Geometry check sheet. Reference: the model listing, model coordinates, mm. A direction names the side the tool comes from. Round coordinates to 2 decimals unless told otherwise and drop trailing zeros. Write each loop counter-clockwise with the first axis right and the second up, starting at its lowest first coordinate (ties: lowest second). Pieces come first, ordered by that corner, then holes. Notation, with made-up numbers: (69.25, 4.5) - (87.25, 4.5) arc R19 ccw to (87.25, 37.5) - close; hole circle Ø9 at (-10.5, 17). An arc over 180 degrees is marked (long way). Return JSON: item names as keys, results as strings.
```python
from build123d import *

# Parameters (mm, degrees)
FILLET1_R   = 0.2
FILLET2_R   = 0.4
HEX_2_DEPTH = 1.6


with BuildPart() as part:
    # BodySke → Base-Revolve (revolve)
    with BuildSketch(Plane.XY):
        Polygon((0, 0), (0, 3.5), (2.8, 3.5), (2.8, 2), (12.41, 2), (12.8, 1.61), (12.8, 0), align=None)
    revolve(axis=Axis((-31.75, 0, 0), (1, 0, 0)))

    # Fillet1
    fillet1_edges = [part.edges().sort_by_distance(p)[0] for p in [
        (2.8, -2, 0),
    ]]
    fillet(fillet1_edges, radius=FILLET1_R)

    # Fillet2
    fillet2_edges = [part.edges().sort_by_distance(p)[0] for p in [
        (0, -3.5, 0),
    ]]
    fillet(fillet2_edges, radius=FILLET2_R)

    # HexSke → Hex 2 (cut)
    with BuildSketch(Plane(origin=(0, 0, 0), x_dir=(0, 0.5, 0.866025404), z_dir=(-1, 0, 0))):
        Polygon((0.866025404, 1.5), (-0.866025404, 1.5), (-1.732050808, 0), (-0.866025404, -1.5), (0.866025404, -1.5), (1.732050808, 0), align=None)
    extrude(amount=-HEX_2_DEPTH, mode=Mode.SUBTRACT)

    # PilotSke → Hex-PreBroach (revolve, cut)
    with BuildSketch(Plane.XY):
        Polygon((0, 1.5), (1.6, 1.5), (1.888675135, 1), (3.3, 1), (3.877350269, 0), (0, 0), align=None)
    revolve(axis=Axis((0, 0, 0), (1, 0, 0)), mode=Mode.SUBTRACT)


solid = part.part
```
(1) Access from +Z, -Z, +X, -X, +Y, -Y to the whole of each face (thin tool, end or side, straight path). Record for faces 4 (the face through (12.8, 0, 0)), 5 (the face through (8, 0, -2)), 6 (the face through (0.789, -1.305, 0.739)).
Response values:
{"face 4": "+Z, -Z, +X, +Y, -Y", "face 5": "+X", "face 6": "-X"}
(2) Section check A-A, the plane x = 5.5. Enter the section's corners in (y, z).
Response values:
{"outline": "circle Ø4 at (0, 0)"}
(3) Gauge pin test, flat ends, axial feed: pin 1 (1 mm diameter, centred on x = 4, z = 0, fed in from +Y); pin 2 (1.6 mm diameter, centred on y = 0, z = 0, fed in from -X); pin 3 (3 mm diameter, centred on x = 7, y = -0.5, fed in from -Z). Record the tip position at first contact, or that the pin passes through.
Response values:
{"pin 1": "stops at y = 2", "pin 2": "stops at x = 3.42", "pin 3": "stops at z = -2"}
(4) Release check for a two-part mould opening along Y. For faces 1 (the face through (0.789, 1.293, 0.761)), 2 (the face through (0, -1.3, -1.3)), 3 (the face through (1.617, 3.233, -1.341)) record: pulls with the +Y half, pulls with the -Y half, needs draft (parallel to the pull), parting line crosses it, or undercut.
Response values:
{"face 1": "undercut", "face 2": "needs draft", "face 3": "parting line crosses it"}
(5) Material ranges on line 1 along Z through (x, y) = (2.4, 0); line 2 along Z through (x, y) = (3, 0); line 3 along X through (y, z) = (-1, 2.25), recorded low to high. Write a range as [from, to].
Response values:
{"line 1": "z = [-3.5, -1], [1, 3.5]", "line 2": "z = [-2, -1], [1, 2]", "line 3": "x = [0, 2.8]"}
